Geometry: final body of the model. Coordinates: model frame, mm. Give positions to 0.01 mm unless a question says otherwise; leave off trailing zeros. Write each loop counter-clockwise with the first axis right and the second up, starting at its lowest first coordinate (ties: lowest second). Pieces come first, ordered by that corner, then holes. Notation, with made-up numbers: (14.5, 62) - (72.5, 62) arc R13 ccw to (72.5, 79) - close; hole circle Ø6 at (-33.75, -21). An arc over 180 degrees is marked (long way). Return JSON: item names as keys, results as strings.
from build123d import *

# Parameters (mm, degrees)
F0_W     = 4.5000037
F0_H     = 13.9999974
F0_W_2   = 4.499991
F0_H_2   = 5.08
F0_W_3   = 4.5000164
F1_DEPTH = 12.7
F2_W     = 94.500065
F2_H     = 24.1599974
F3_DEPTH = 6.35
F4_R     = 2.54


with BuildPart() as f1:
    # F0 (on Top) → F1 (new body)
    with BuildSketch(Plane.XY):
        Polygon((-64.6874586299, 19.0799974), (-60.1874549299, 19.0799974), (-60.1874549299, 24.1599974), (-69.1874623299, 24.1599974), (-69.1874623299, 19.0799974), align=None)
        with Locations((-66.9374604799, 12.0799987)):
            Rectangle(F0_W, F0_H)
        Polygon((-69.1874623299, 0), (-60.1874549299, 0), (-60.1874549299, 5.08), (-64.6874586299, 5.08), (-69.1874623299, 5.08), align=None)
        Polygon((-60.1874549299, 0), (-51.1874475299, 0), (-51.1874475299, 5.08), (-55.6874512299, 5.08), (-60.1874549299, 5.08), align=None)
        with Locations((-57.9374530799, 12.0799987)):
            Rectangle(F0_W, F0_H)
        Polygon((-55.6874512299, 19.0799974), (-51.1874475299, 19.0799974), (-51.1874475299, 24.1599974), (-60.1874549299, 24.1599974), (-60.1874549299, 19.0799974), align=None)
        Polygon((-46.6874438299, 19.0799974), (-42.1874401299, 19.0799974), (-42.1874401299, 24.1599974), (-51.1874475299, 24.1599974), (-51.1874475299, 19.0799974), align=None)
        with Locations((-48.9374456799, 12.0799987)):
            Rectangle(F0_W, F0_H)
        Polygon((-51.1874475299, 0), (-42.1874401299, 0), (-42.1874401299, 5.08), (-46.6874438299, 5.08), (-51.1874475299, 5.08), align=None)
        Polygon((-42.1874401299, 0), (-33.1874327299, 0), (-33.1874327299, 5.08), (-37.6874364299, 5.08), (-42.1874401299, 5.08), align=None)
        with Locations((-39.9374382799, 12.0799987)):
            Rectangle(F0_W, F0_H)
        Polygon((-37.6874364299, 19.0799974), (-33.1874327299, 19.0799974), (-33.1874327299, 24.1599974), (-42.1874401299, 24.1599974), (-42.1874401299, 19.0799974), align=None)
        Polygon((-28.6874290299, 19.0799974), (-24.1874253299, 19.0799974), (-24.1874253299, 24.1599974), (-33.1874327299, 24.1599974), (-33.1874327299, 19.0799974), align=None)
        with Locations((-30.9374308799, 12.0799987)):
            Rectangle(F0_W, F0_H)
        Polygon((-33.1874327299, 0), (-24.1874253299, 0), (-24.1874253299, 5.08), (-28.6874290299, 5.08), (-33.1874327299, 5.08), align=None)
        with Locations((-21.9374298299, 12.0799987)):
            Rectangle(F0_W_2, F0_H)
        with Locations((-21.9374298299, 2.54)):
            Rectangle(F0_W_2, F0_H_2)
        with Locations((-17.4374261299, 2.54)):
            Rectangle(F0_W_3, F0_H_2)
        Polygon((-24.1874253299, 24.1599974), (-24.1874253299, 19.0799974), (-19.6874343299, 19.0799974), (-15.1874179299, 19.0799974), (-15.1874179299, 24.1599974), align=None)
        Polygon((-15.1874179299, 5.08), (-15.1874179299, 0), (-6.1874105299, 0), (-6.1874105299, 5.08), (-10.6874142299, 5.08), align=None)
        with Locations((-12.9374160799, 12.0799987)):
            Rectangle(F0_W, F0_H)
        Polygon((-15.1874179299, 24.1599974), (-15.1874179299, 19.0799974), (-10.6874142299, 19.0799974), (-6.1874105299, 19.0799974), (-6.1874105299, 24.1599974), align=None)
        Polygon((-6.1874105299, 24.1599974), (-6.1874105299, 19.0799974), (-1.6874068299, 19.0799974), (2.8125968701, 19.0799974), (2.8125968701, 24.1599974), align=None)
        with Locations((-3.9374086799, 12.0799987)):
            Rectangle(F0_W, F0_H)
        Polygon((-6.1874105299, 5.08), (-6.1874105299, 0), (2.8125968701, 0), (2.8125968701, 5.08), (-1.6874068299, 5.08), align=None)
        Polygon((2.8125968701, 5.08), (2.8125968701, 0), (11.8126042701, 0), (11.8126042701, 5.08), (7.3126005701, 5.08), align=None)
        with Locations((5.0625987201, 12.0799987)):
            Rectangle(F0_W, F0_H)
        Polygon((2.8125968701, 24.1599974), (2.8125968701, 19.0799974), (7.3126005701, 19.0799974), (11.8126042701, 19.0799974), (11.8126042701, 24.1599974), align=None)
        Polygon((11.8126042701, 24.1599974), (11.8126042701, 19.0799974), (16.3126079701, 19.0799974), (20.8126116701, 19.0799974), (20.8126116701, 24.1599974), align=None)
        with Locations((14.0626061201, 12.0799987)):
            Rectangle(F0_W, F0_H)
        Polygon((11.8126042701, 5.08), (11.8126042701, 0), (20.8126116701, 0), (20.8126116701, 5.08), (16.3126079701, 5.08), align=None)
        Polygon((20.8126116701, 5.08), (20.8126116701, 0), (25.3126026701, 0), (25.3126026701, 24.1599974), (20.8126116701, 24.1599974), (20.8126116701, 19.0799974), align=None)
    extrude(amount=F1_DEPTH)

    # F2 (on face) → F3 (join)
    with BuildSketch(Plane(origin=(0, 0, 0), x_dir=(1, 0, 0), z_dir=(0, 0, -1))):
        with Locations((-21.9374298299, -12.0799987)):
            Rectangle(F2_W, F2_H)
    extrude(amount=F3_DEPTH)

    # F4
    f4_edges = [f1.edges().sort_by_distance(p)[0] for p in [
        (-21.93743, 24.159997, 12.7),
        (-21.93743, 0, 12.7),
        (-69.187462, 12.079999, 12.7),
        (25.312603, 12.079999, 12.7),
    ]]
    fillet(f4_edges, radius=F4_R)


solid = f1.part
Q1. Mould query, pull axis X, two halves, no side actions, for faces 1 (the flat face through (-6.187, 12, 6)), 2 (the flat face through (-23, 12, -6.35)), 3 (the cylindrical face through (24.588, 12.249, 11.936)). Classes: pulls with the +X half, pulls with the -X half, needs draft (parallel to the pull), parting line crosses it, or undercut.
Answer key:
{"face 1": "undercut", "face 2": "needs draft", "face 3": "pulls with the +X half"}
Q2. Pin query (flat end, axial travel): P1, Ø1.4, axis at x = -62.5, y = 9, coming from the +Z side. Return the tip coordinate at first contact, or that it passes through.
Answer key:
{"P1": "stops at z = 0"}
Q3. Section query B-B, the plane z = 9. Count the separate pieces of the cut face and the enclosed holes in it, plus the area to 3 significant figures.
Answer key:
{"separate pieces": "1", "enclosed holes": "10", "area": "1,650 mm^2"}
Q4. Material intervals for probe 1 along Y at (x, z) = (-19, 1); probe 2 along Z at (x, y) = (-52, 14.75); probe 3 along Y at (x, z) = (-21, 11), sorted ascending. Write a range as [from, to].
Answer key:
{"probe 1": "y = [0, 5.08], [19.08, 24.16]", "probe 2": "z = [-6.35, 0]", "probe 3": "y = [0.14, 24.02]"}
Q5. Section query A-A, the plane x = -25.5. Return the cut outline in (y, z), plus the area to 3 significant figures.
Answer key:
{"outline": "(0, -6.35) - (24.16, -6.35) - (24.16, 10.16) arc R2.54 ccw to (21.62, 12.7) - (19.08, 12.7) - (19.08, 0) - (5.08, 0) - (5.08, 12.7) - (2.54, 12.7) arc R2.54 ccw to (0, 10.16) - close", "area": "280 mm^2"}
